Here's how the part is built. I have some questions about the finished solid (model axes, mm). A direction names the side the tool comes from. Coordinates: 2 decimals unless noted, no trailing zeros. Loops run counter-clockwise (first coordinate to the right, second up) from the corner with the lowest first, then second, coordinate; pieces in that order, holes last. Notation, with made-up numbers: (62.5, 20.5) - (70.5, 20.5) arc R27 ccw to (70.5, 42.5) - close; hole circle Ø6 at (1.5, -7.75). An arc over 180 degrees is marked (long way). Use a Markdown table: item, result.
```python
from build123d import *

# Parameters (mm, degrees)
RESSALTO_EXTRUS_O1_DEPTH                            = 80
CHANFRO2_SIZE                                       = 5
ESCAREADO_PARA_PARAFUSO_ALLEN_SEXTAVADO_D           = 6.6
ESCAREADO_PARA_PARAFUSO_ALLEN_SEXTAVADO_CSINK_D     = 13.44
ESCAREADO_PARA_PARAFUSO_ALLEN_SEXTAVADO_CSINK_ANGLE = 90


with BuildPart() as part:
    # Esboço1 → Ressalto-extrusão1 (new body)
    with BuildSketch(Plane(origin=(0, 0, 0), x_dir=(1, 0, 0), z_dir=(0, 1, 0))):
        Polygon((0, 0), (0, 7), (-135.225243436, 7), (-138, 4.225243436), (-138, -0.135644581), (-135.135644581, -3), (-60, -3), (-60, 0), align=None)
    extrude(amount=RESSALTO_EXTRUS_O1_DEPTH)

    # Chanfro2
    chanfro2_edges = [part.edges().sort_by_distance(p)[0] for p in [
        (-30, 80, 0),
    ]]
    chamfer(chanfro2_edges, length=CHANFRO2_SIZE)

    # Escareado para parafuso Allen sextavado escareado de M62 (through all)
    with Locations(Plane.XY):
        with Locations((-18, 63), (-50, 53), (-18, 28), (-50, 8)):
            CounterSinkHole(ESCAREADO_PARA_PARAFUSO_ALLEN_SEXTAVADO_D / 2, ESCAREADO_PARA_PARAFUSO_ALLEN_SEXTAVADO_CSINK_D / 2, counter_sink_angle=ESCAREADO_PARA_PARAFUSO_ALLEN_SEXTAVADO_CSINK_ANGLE)


solid = part.part
```
Q1. If we mould it in two halves opening along X, with no side actions, what happens to faces 1 (the face through (-98, 39, 3)), 2 (the face through (0, 39, -3)), 3 (the face through (-47.57, 55.23, -5.24))? For each: pulls with the +X half, pulls with the -X half, needs draft (parallel to the pull), parting line crosses it, or undercut.
Check values:
| item | result |
|---|---|
| face 1 | needs draft |
| face 2 | pulls with the +X half |
| face 3 | undercut |
Q2. Will these pins go through, and if not, where does the flat tip stop? P1, Ø8, axis at x = -41, y = 43, coming from the +Z side; P2, Ø1.5, axis at x = -21, z = -1.5, coming from the +Y side; P3, Ø1.5, axis at y = 54, z = 2, coming from the -X side.
Check values:
| item | result |
|---|---|
| P1 | z = 0 |
| P2 | y = 77.25 |
| P3 | x = -136.89 |
Q3. Which directions (+Z, -Z, +X, -X, +Y, -Y) give clear straight access to the entire face, cutting with the end or side of a thin tool? Please do faces 4 (the face through (-30, 78, -3)), 5 (the face through (-30, 37, 0)), 6 (the face through (-21.31, 29.04, -3.25)).
Check values:
| item | result |
|---|---|
| face 4 | +Z, +X, +Y |
| face 5 | +Z, +X, +Y, -Y |
| face 6 | +Z |
Q4. I want a section at A-A, the plane x = -18. Write out the boundary of the cut face in (y, z).
Check values:
| item | result |
|---|---|
| outline | (0, -7) - (24.7, -7) - (24.7, -3.42) - (21.28, 0) - (0, 0) - close; (31.3, -7) - (59.7, -7) - (59.7, -3.42) - (56.28, 0) - (34.72, 0) - (31.3, -3.42) - close; (66.3, -7) - (80, -7) - (80, -5) - (75, 0) - (69.72, 0) - (66.3, -3.42) - close |
Q5. Please list where these lines run through material, in increasing order: L1, parallel to Y at x = -50, z = -5.55; L2, parallel to Y at x = -18, z = -5.15; L3, parallel to Z at x = -37, y = 49. Write a range as from..to.
Check values:
| item | result |
|---|---|
| L1 | 0..4.7, 11.3..49.7, 56.3..80 |
| L2 | 0..24.7, 31.3..59.7, 66.3..80 |
| L3 | -7..0 |
Q6. I want a section at C-C, the plane y = 45. Write out the boundary of the cut face in (x, z), then the cut area to 3 significant figures.
Check values:
| item | result |
|---|---|
| outline | (-138, -4.23) - (-135.23, -7) - (0, -7) - (0, 0) - (-60, 0) - (-60, 3) - (-135.14, 3) - (-138, 0.14) - close |
| area | 1,190 mm^2 |
Q7. I want a section at D-D, the plane x = -38. Write out the boundary of the cut face in (y, z), then the cut area to 4 significant figures.
Check values:
| item | result |
|---|---|
| outline | (0, -7) - (80, -7) - (80, -5) - (75, 0) - (0, 0) - close |
| area | 547.5 mm^2 |
Q8. I want a section at B-B, the plane y = 63. Write out the boundary of the cut face in (x, z).
Check values:
| item | result |
|---|---|
| outline | (-138, -4.23) - (-135.23, -7) - (-21.3, -7) - (-21.3, -3.42) - (-24.72, 0) - (-60, 0) - (-60, 3) - (-135.14, 3) - (-138, 0.14) - close; (-14.7, -7) - (0, -7) - (0, 0) - (-11.28, 0) - (-14.7, -3.42) - close |
